Model file for the job. Use its own axes, mm. Face numbers are marked on the shaded views. Round coordinates to 2 decimals unless told otherwise and drop trailing zeros. Loops run counter-clockwise (first coordinate to the right, second up) from the corner with the lowest first, then second, coordinate; pieces in that order, holes last.
from build123d import *

# Parameters (mm, degrees)
SKETCH1_W          = 141
SKETCH1_H          = 104.7
EXTRUDE1_DEPTH     = 6.2
SKETCH4_W          = 160
SKETCH4_H          = 109
EXTRUDE2_DEPTH     = 0.3
SKETCH5_R          = 1.75
CUT_EXTRUDE1_DEPTH = 0.3
SKETCH3_W          = 122
SKETCH3_H          = 92
CUT_EXTRUDE4_DEPTH = 0.2


with BuildPart() as part:
    # Sketch1 → Extrude1 (new body)
    with BuildSketch(Plane.XY):
        with Locations((70.5, -52.35)):
            Rectangle(SKETCH1_W, SKETCH1_H)
    extrude(amount=EXTRUDE1_DEPTH)

    # Sketch4 → Extrude2 (add)
    with BuildSketch(Plane(origin=(0, 0, 0), x_dir=(-1, 0, 0), z_dir=(0, 0, -1))):
        with Locations((-69, -52.35)):
            Rectangle(SKETCH4_W, SKETCH4_H)
    extrude(amount=EXTRUDE2_DEPTH)

    # Sketch5 → Cut-Extrude1 (cut)
    with BuildSketch(Plane.XY):
        with Locations((145, -1.85)):
            Circle(SKETCH5_R)
        with Locations((145, -102.85)):
            Circle(SKETCH5_R)
        with Locations((-7, -1.85)):
            Circle(SKETCH5_R)
        with Locations((-7, -102.85)):
            Circle(SKETCH5_R)
    extrude(amount=-CUT_EXTRUDE1_DEPTH, mode=Mode.SUBTRACT)

    # Sketch3 → Cut-Extrude4 (cut)
    with BuildSketch(Plane.XY.offset(6.2)):
        with Locations((74.985806668, -52.998526077)):
            Rectangle(SKETCH3_W, SKETCH3_H)
    extrude(amount=-CUT_EXTRUDE4_DEPTH, mode=Mode.SUBTRACT)


solid = part.part
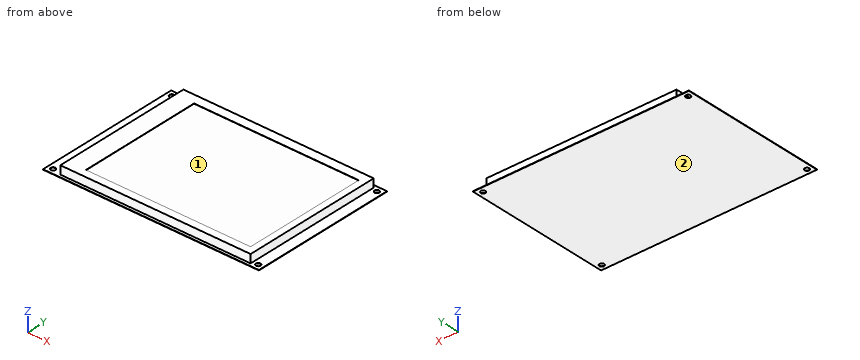
Q1. Flat gauge pins, fed straight in: P1, Ø3, axis at x = 45, z = 3, coming from the -Y side; P2, Ø10, axis at x = 124, y = -14.5, coming from the +Z side; P3, Ø12, axis at x = 15, y = -80, coming from the +Z side; P4, Ø1.5, axis at x = 71, z = 4.5, coming from the +Y side. Where does each tip first touch, or does it go through?
Q2. Slice it at C-C on y = -89.5. Give the cut face in (x, z).
Q3. Probe line 1 (Y direction, x = 145, z = -0.15); line 2 (X direction, y = -100, z = 4); line 3 (Z direction, x = 124.5, y = -55). List the from-to ranges inside material, lowest first.
Q4. Slice it at D-D on x = 109.5. Give the cut face in (y, z), plus the area to 3 significant figures.
Q5. Slice it at B-B on x = 145. Give the cut face in (y, z).
Q6. Slice it at A-A on y = -1.85. Give the cut face in (x, z), plus the area to 3 significant figures.
Q7. Pull direction Y, two halves, no side cores. Call the marked faces 1 and 2: pulls with the +Y half, pulls with the -Y half, needs draft (parallel to the pull), parting line crosses it, or undercut.
Reply:
1. P1: stops at y = -104.7
1. P2: stops at z = 6
1. P3: stops at z = 6.2
1. P4: stops at y = 0
2. outline: (-11, -0.3) - (149, -0.3) - (149, 0) - (141, 0) - (141, 6.2) - (135.99, 6.2) - (135.99, 6) - (13.99, 6) - (13.99, 6.2) - (0, 6.2) - (0, 0) - (-11, 0) - close
3. line 1: y = -106.85 to -104.6, -101.1 to -3.6, -0.1 to 2.15
3. line 2: x = 0 to 141
3. line 3: z = -0.3 to 6
4. outline: (-106.85, -0.3) - (2.15, -0.3) - (2.15, 0) - (0, 0) - (0, 6.2) - (-7, 6.2) - (-7, 6) - (-99, 6) - (-99, 6.2) - (-104.7, 6.2) - (-104.7, 0) - (-106.85, 0) - close
4. area: 663 mm2
5. outline: (-106.85, -0.3) - (-104.6, -0.3) - (-104.6, 0) - (-106.85, 0) - close; (-101.1, -0.3) - (-3.6, -0.3) - (-3.6, 0) - (-101.1, 0) - close; (-0.1, -0.3) - (2.15, -0.3) - (2.15, 0) - (-0.1, 0) - close
6. outline: (-11, -0.3) - (-8.75, -0.3) - (-8.75, 0) - (-11, 0) - close; (-5.25, -0.3) - (143.25, -0.3) - (143.25, 0) - (141, 0) - (141, 6.2) - (0, 6.2) - (0, 0) - (-5.25, 0) - close; (146.75, -0.3) - (149, -0.3) - (149, 0) - (146.75, 0) - close
6. area: 920 mm2
7. face 1: undercut
7. face 2: needs draft
